Can you work these out from the model? Positions are in its coordinate system, mm. Face numbers are marked on the shaded views. A direction names the side the tool comes from. Give positions to 0.01 mm unless a question says otherwise; leave off trailing zeros. Loops run counter-clockwise (first coordinate to the right, second up) from the corner with the lowest first, then second, coordinate; pieces in that order, holes last. Notation, with made-up numbers: (61, 24.5) -> (107, 24.5) arc R26 ccw to (107, 43.5) -> close; hole circle Ø6 at (23.25, 23.5). An arc over 180 degrees is marked (long way). Return JSON: item names as keys, results as strings. Group by question number.
Q1. Will these pins go through, and if not, where does the flat tip stop? pin 1 (1.5 mm diameter, centred on x = 3.5, z = 21, fed in from -Y); pin 2 (2.5 mm diameter, centred on x = 0.5, y = -1, fed in from -Z); pin 3 (1.5 mm diameter, centred on y = 2.5, z = 5.5, fed in from -X).
Q2. Suppose I cut it at C-C, the plane z = 7.5. Please give me the cut outline in (x, y), and give its area (3 significant figures).
Q3. Suppose I cut it at A-A, the plane x = 0. Please give me the cut outline in (y, z).
Q4. Thinking about a two-plate mould opening in Z: for the marked faces 5, 6 and 7, which applies, pulls with the +Z half, pulls with the -Z half, needs draft (parallel to the pull), parting line crosses it, or undercut?
Q5. Suppose I cut it at D-D, the plane y = -4.5. Please give me the cut outline in (x, z), and give its area (3 significant figures).
Q6. Suppose I cut it at B-B, the plane y = 0. Please give me the cut outline in (x, z), and give its area (3 significant figures).
Q7. Which directions (+Z, -Z, +X, -X, +Y, -Y) give clear straight access to the entire face, cutting with the end or side of a thin tool? Please do the marked faces 1, 2, 3 and 4.
Q8. I need wall thicknesses on line 1 along Z through (x, y) = (0, -4.2); line 2 along Z through (x, y) = (1, -6); line 3 along Z through (x, y) = (0, -3.15). Which ranges of each line are inside material? Lowest first, please. Write a range as [from, to].
```python
from build123d import *

# Parameters (mm, degrees)
ESBO_O1_R                 = 7.5
RESSALTO_EXTRUS_O1_DEPTH  = 25
ESBO_O2_R                 = 2.55
CORTE_EXTRUS_O1_DEPTH     = 5
CORTE_EXTRUS_O2_START     = 7
CORTE_EXTRUS_O2_OUTLINE_R = 3.706811579
CORTE_EXTRUS_O2_DEPTH     = 18
ESBO_O3_R                 = 1.5
CORTE_EXTRUS_O3_DEPTH     = 18


# Read off the part's stored shape, not the designer's step: Corte-extrusão2
with BuildPart() as part:
    # Esboço1 → Ressalto-extrusão1 (new body)
    with BuildSketch(Plane.XY):
        Circle(ESBO_O1_R)
    extrude(amount=RESSALTO_EXTRUS_O1_DEPTH)

    # Esboço2 → Corte-extrusão1 (cut)
    with BuildSketch(Plane.XY):
        Circle(ESBO_O2_R)
    extrude(amount=CORTE_EXTRUS_O1_DEPTH, mode=Mode.SUBTRACT)

    # Corte-extrusão2 outline → Corte-extrusão2 (cut)
    with BuildSketch(Plane.XY.offset(CORTE_EXTRUS_O2_START)):
        Circle(CORTE_EXTRUS_O2_OUTLINE_R)
    extrude(amount=CORTE_EXTRUS_O2_DEPTH, mode=Mode.SUBTRACT)

    # Esboço3 → Corte-extrusão3 (cut)
    with BuildSketch(Plane(origin=(0, 0, 0), x_dir=(1, 0, 0), z_dir=(0, 1, 0))):
        with Locations(Location((0, -2.967761403, 0), (0, 0, 270))):
            Circle(ESBO_O3_R)
        with Locations(Location((0, -22.5, 0), (0, 0, 270))):
            Circle(ESBO_O3_R)
    extrude(amount=-CORTE_EXTRUS_O3_DEPTH, mode=Mode.SUBTRACT)


solid = part.part
```
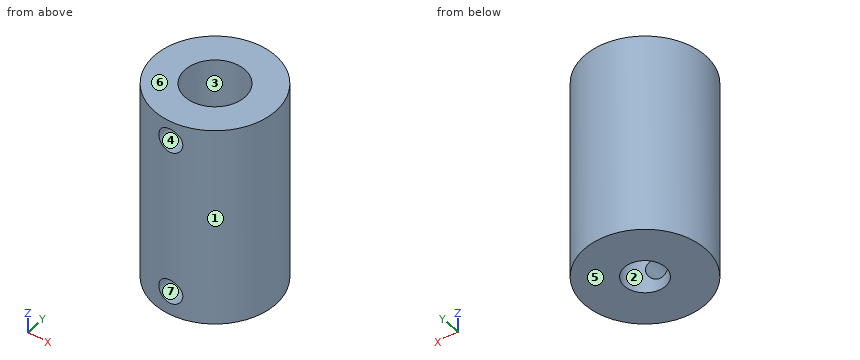
Ans:
{
 "1": {"pin 1": "stops at y = -6.98", "pin 2": "stops at z = 5", "pin 3": "stops at x = -7.29"},
 "2": {"outline": "circle Ø15 at (0, 0); hole circle Ø7.41 at (0, 0)", "area": "134 mm^2"},
 "3": {"outline": "(-7.5, 0) -> (-2.55, 0) -> (-2.55, 1.47) -> (-7.5, 1.47) -> close; (-7.5, 4.47) -> (-2.55, 4.47) -> (-2.55, 5) -> (2.55, 5) -> (2.55, 0) -> (7.5, 0) -> (7.5, 25) -> (3.71, 25) -> (3.71, 7) -> (-3.71, 7) -> (-3.71, 21) -> (-7.5, 21) -> close; (-7.5, 24) -> (-3.71, 24) -> (-3.71, 25) -> (-7.5, 25) -> close"},
 "4": {"face 5": "pulls with the -Z half", "face 6": "pulls with the +Z half", "face 7": "undercut"},
 "5": {"outline": "(-6, 0) -> (6, 0) -> (6, 25) -> (-6, 25) -> close; hole circle Ø3 at (0, 2.97); hole circle Ø3 at (0, 22.5)", "area": "286 mm^2"},
 "6": {"outline": "(-7.5, 0) -> (-2.55, 0) -> (-2.55, 5) -> (2.55, 5) -> (2.55, 0) -> (7.5, 0) -> (7.5, 25) -> (3.71, 25) -> (3.71, 7) -> (-3.71, 7) -> (-3.71, 25) -> (-7.5, 25) -> close", "area": "216 mm^2"},
 "7": {"face 1": "+Z, -Z", "face 2": "-Z", "face 3": "+Z", "face 4": "-Y"},
 "8": {"line 1": "z = [0, 1.47], [4.47, 21], [24, 25]", "line 2": "z = [0, 1.85], [4.09, 21.38], [23.62, 25]", "line 3": "z = [0, 1.47], [4.47, 7]"}
}
